from build123d import *

# Parameters (mm, degrees)
F0_W     = 25.4
F0_H     = 12.065
F1_DEPTH = 0.3048


with BuildPart() as f1:
    # F0 (on Top) → F1 (new body)
    with BuildSketch(Plane.XY):
        with Locations((0, -0.635)):
            Rectangle(F0_W, F0_H)
        with BuildLine():
            Line((52.643894, 19.802554), (12.7, 5.3975))
            Line((12.7, 5.3975), (12.7, -6.6675))
            Line((12.7, -6.6675), (52.643894, -21.072554))
            ThreePointArc((52.643894, -21.072554), (55.54594, -20.683957), (56.896, -18.085839))
            Line((56.896, -18.085839), (56.896, -0.635))
            Line((56.896, -0.635), (56.896, 16.815839))
            ThreePointArc((56.896, 16.815839), (55.54594, 19.413957), (52.643894, 19.802554))
        make_face()
        with BuildLine():
            Line((-12.7, -6.6675), (-12.7, 5.3975))
            Line((-12.7, 5.3975), (-52.629368, 20.017363))
            ThreePointArc((-52.629368, 20.017363), (-55.539611, 19.638479), (-56.896, 17.035927))
            Line((-56.896, 17.035927), (-56.896, -0.391439))
            Line((-56.896, -0.391439), (-56.896, -17.86567))
            ThreePointArc((-56.896, -17.86567), (-55.552281, -20.459323), (-52.658498, -20.857612))
            Line((-52.658498, -20.857612), (-12.7, -6.6675))
        make_face()
    extrude(amount=F1_DEPTH)


solid = f1.part
Geometry check sheet. Reference: the model listing, model coordinates, mm. A direction names the side the tool comes from. Round coordinates to 2 decimals unless told otherwise and drop trailing zeros. Order: outer loops, then holes, each group sorted by start corner. A loop starts at its lowest first (then second) coordinate and runs counter-clockwise, first axis right, second up. Notation, with made-up numbers: (16.5, 2) -> (26.5, 2) arc R31 cw to (26.5, 32) -> close; hole circle Ø5 at (42, 43). An arc over 180 degrees is marked (long way). Use one line per item in the form item = value.
1. Set-up check for faces 1 (the face through (55.58, 19.39, 0.15)), 2 (the face through (-32.959, -13.862, 0.15)): record each of +Z, -Z, +X, -X, +Y, -Y from which the full face is reachable in a straight line by a thin tool's end or side.
Working result:
face_1 = +Z, -Z, +Y
face_2 = +Z, -Z, -Y
2. Cross-section at A-A, the plane y = 14. Enter the section's corners in (x, z), plus the area to 3 significant figures.
Working result:
outline = (-56.9, 0) -> (-36.19, 0) -> (-36.19, 0.3) -> (-56.9, 0.3) -> close; (36.55, 0) -> (56.9, 0) -> (56.9, 0.3) -> (36.55, 0.3) -> close
area = 12.5 mm^2
3. Mould release check, pull along X, two halves, no side actions. Record for faces 3 (the face through (55.51, -20.71, 0.15)), 4 (the face through (-1, 0, 0.305)), 5 (the face through (-55.587, -20.435, 0.15)), 6 (the face through (32.39, -13.77, 0.15)): pulls with the +X half, pulls with the -X half, needs draft (parallel to the pull), parting line crosses it, or undercut.
Working result:
face_3 = parting line crosses it
face_4 = needs draft
face_5 = undercut
face_6 = undercut
4. Cross-section at D-D, the plane x = 17.5. Enter the section's corners in (y, z), plus the area to 3 significant figures.
Working result:
outline = (-8.4, 0) -> (7.13, 0) -> (7.13, 0.3) -> (-8.4, 0.3) -> close
area = 4.73 mm^2
5. Cross-section at C-C, the plane y = 18.5. Enter the section's corners in (x, z).
Working result:
outline = (-56.54, 0) -> (-48.49, 0) -> (-48.49, 0.3) -> (-56.54, 0.3) -> close; (49.03, 0) -> (56.41, 0) -> (56.41, 0.3) -> (49.03, 0.3) -> close
6. Scan lines: line 1 along Y through (x, z) = (5.5, 0.15); line 2 along Y through (x, z) = (13, 0.1). Record each from-to range of solid material in increasing order. Write a range as from..to.
Working result:
line_1 = -6.67..5.4
line_2 = -6.78..5.51
